Autodesk Inventor part; units mm, degrees
ref_plane "YZ Plane" through (0, 0, 0) normal (1, 0, 0) x (0, 1, 0)
ref_plane "XZ Plane" through (0, 0, 0) normal (0, 1, 0) x (-1, 0, 0)
ref_plane "XY Plane" through (0, 0, 0) normal (0, 0, 1) x (1, 0, 0)
sketch "スケッチ2" plane through (0, 0, 0) normal (0, 1, 0) x (-1, 0, 0)
  line L0 (0, 1.5) -> (-0.75, 1.5)
  line L1 (-0.75, 2.25) -> (-0.75, 3.75)
  line L2 (-0.75, 3.75) -> (0, 3.75)
  line L3 (0, 3.75) -> (0, 1.5)
  line L4 (-0.75, 1.5) -> (-3, 1.5)
  line L5 (-3, 1.5) -> (-3, 2.1923)
  line L6 (0, 0) -> (-4.3872, 0)
  line L7 (-3, 2.1923) -> (-2.9, 2.25)
  line L8 (-2.9, 2.25) -> (-0.75, 2.25)
  dimension "d0" = 3.75
  dimension "d2" = 1.5
  dimension "d3" = 0.75
  dimension "d4" = 3
  dimension "d5" = 30
  dimension "d6" = 2.25
  dimension "d7" = 0.1
  dimension "d8" = 0
revolve "回転1" add sketch "スケッチ2" angle 360 about axis through (0, 0, 0) along (1, 0, 0)
properties part number "GFM-0304-03" material "PAEK 樹脂"
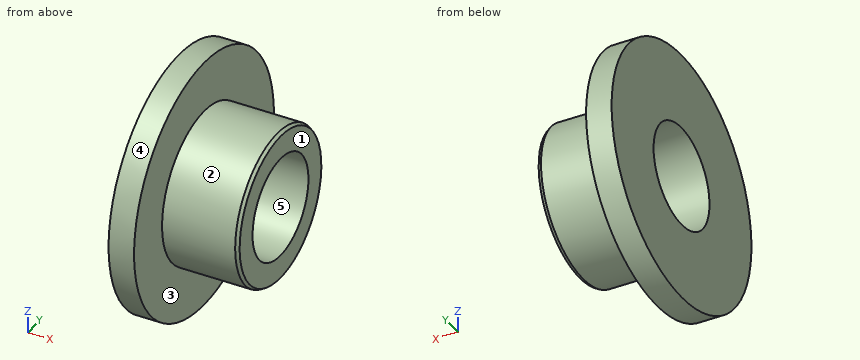
CAD build for the part. Positions are in the model's coordinates, mm. Face numbers are marked on the shaded views. A direction names the side the tool comes from. Give positions to 0.01 mm unless a question says otherwise; leave off trailing zeros. Write each loop counter-clockwise with the first axis right and the second up, starting at its lowest first coordinate (ties: lowest second). Pieces come first, ordered by that corner, then holes. Notation, with made-up numbers: (75, 60.25) -> (94, 60.25) arc R21 cw to (94, 70.25) -> close; hole circle Ø5 at (24, 17). An arc over 180 degrees is marked (long way). Return JSON: item names as keys, results as strings.
Item 1: Band-saw the part on C-C (x = 0.3). List the corners of the cut face in (y, z), then the cut area to 3 significant figures.
Answer below:
{"outline": "circle Ø7.5 at (0, 0); hole circle Ø3 at (0, 0)", "area": "37.1 mm2"}
Item 2: Band-saw the part on A-A (z = 0). List the corners of the cut face in (x, y).
Answer below:
{"outline": "(0, -3.75) -> (0.75, -3.75) -> (0.75, -2.25) -> (2.9, -2.25) -> (3, -2.19) -> (3, -1.5) -> (0, -1.5) -> close; (0, 1.5) -> (3, 1.5) -> (3, 2.19) -> (2.9, 2.25) -> (0.75, 2.25) -> (0.75, 3.75) -> (0, 3.75) -> close"}
Item 3: Band-saw the part on D-D (x = 1.35). List the corners of the cut face in (y, z).
Answer below:
{"outline": "circle Ø4.5 at (0, 0); hole circle Ø3 at (0, 0)"}
Item 4: Tool access for the marked faces 1 and 2: list every direction of +Z, -Z, +X, -X, +Y, -Y with a clear straight run to the whole face (end or side of a thin tool).
Answer below:
{"face 1": "+Z, -Z, +X, +Y, -Y", "face 2": "+X"}
Item 5: Two-plate mould, pull along Z, no slides. Class the marked faces 3, 4 and 5: +Z half, -Z half, draft (parallel to the pull), parting line (faces both ways), or undercut.
Answer below:
{"face 3": "draft", "face 4": "parting line", "face 5": "undercut"}
Item 6: Drill centre lines: probe 1 along Y at (x, z) = (1.35, 0); probe 2 along X at (y, z) = (2.25, -1). Where is each one in solid material? Low to high.
Answer below:
{"probe 1": "y = -2.25 to -1.5, 1.5 to 2.25", "probe 2": "x = 0 to 0.75"}
